from build123d import *

# Parameters (mm, degrees)
SKETCH3_W           = 41
SKETCH3_H           = 20.5
BOSS_EXTRUDE1_DEPTH = 37
SKETCH5_W           = 12
SKETCH5_H           = 8
BOSS_EXTRUDE2_DEPTH = 5
SKETCH6_R           = 1.5
CUT_EXTRUDE1_DEPTH  = 30


with BuildPart() as part:
    # Sketch3 → Boss-Extrude1 (new body)
    with BuildSketch(Plane(origin=(0, 0, 0), x_dir=(1, 0, 0), z_dir=(0, 1, 0))):
        with Locations((20.5, 10.25)):
            Rectangle(SKETCH3_W, SKETCH3_H)
    extrude(amount=BOSS_EXTRUDE1_DEPTH)

    # Sketch5 → Boss-Extrude2 (add)
    with BuildSketch(Plane(origin=(0, 37, 0), x_dir=(1, 0, 0), z_dir=(0, 1, 0))):
        with Locations((31.406806077, 9.876249369)):
            Rectangle(SKETCH5_W, SKETCH5_H)
    extrude(amount=BOSS_EXTRUDE2_DEPTH)

    # Sketch6 → Cut-Extrude1 (cut)
    with BuildSketch(Plane(origin=(0, 42, 0), x_dir=(1, 0, 0), z_dir=(0, 1, 0))):
        with Locations((34.09544318, 9.783255032)):
            Circle(SKETCH6_R)
    extrude(amount=-CUT_EXTRUDE1_DEPTH, mode=Mode.SUBTRACT)


solid = part.part
Check sheet for the modelled part. Datum: model origin and axes. Units: mm. A direction names the side the tool comes from. Give positions to 0.01 mm unless a question says otherwise; leave off trailing zeros. Loops run counter-clockwise (first coordinate to the right, second up) from the corner with the lowest first, then second, coordinate; pieces in that order, holes last. Notation, with made-up numbers: M -4.75,8.5 L 17.25,8.5 A20 ccw 17.25,24.5 Z; hole C 50.25,72 d1. An arc over 180 degrees is marked long. Use a Markdown table: item, result. Add a question column.
Q1. Scan lines: line 1 along X through (y, z) = (39, -12); line 2 along Y through (x, z) = (10, -14); line 3 along Z through (x, y) = (33.5, 18). Record each from-to range of solid material in increasing order. Write a range as [from, to].
Q2. Sectioned sample at B-B, the plane z = -13.25. Record the cut outline in (x, y).
Q3. Sectioned sample at D-D, the plane x = 3. Record the cut outline in (y, z), then the cut area to 4 significant figures.
Q4. Sectioned sample at C-C, the plane y = 38.5. Record the cut outline in (x, z).
Q5. Tool access check on faces 1 (the flat face through (31, 39, -13.876)), 2 (the flat face through (37.407, 39, -10)), 3 (the flat face through (34, 12, -10)), 4 (the flat face through (31, 39, -5.876)). Record the directions out of +Z, -Z, +X, -X, +Y, -Y that give a thin tool (end or side, any length) a straight path to the whole face; none if there is none.
Q6. Sectioned sample at A-A, the plane x = 30.5. Record the cut outline in (y, z).
Q7. Go/stop test with flat-tipped pins: pin 1 (1 mm diameter, centred on x = 28.5, z = -15, fed in from +Y); pin 2 (1.5 mm diameter, centred on y = 39, z = -9.5, fed in from -X); pin 3 (1.5 mm diameter, centred on y = 39, z = -11.5, fed in from +X). Record where each tip stops, or that it passes through.
Q8. Mould release check, pull along Z, two halves, no side actions. Record for faces 5 (the cylindrical face through (32.905, 27.21, -8.871)), 6 (the flat face through (20, 18, 0)), 7 (the flat face through (25.407, 39, -10)): pulls with the +Z half, pulls with the -Z half, needs draft (parallel to the pull), parting line crosses it, or undercut.
Verdict:
| question | item | result |
|---|---|---|
| 1 | line 1 | [25.41, 37.41] |
| 1 | line 2 | [0, 37] |
| 1 | line 3 | [-20.5, -11.16], [-8.41, 0] |
| 2 | outline | M 0,0 L 41,0 L 41,37 L 37.41,37 L 37.41,42 L 25.41,42 L 25.41,37 L 0,37 Z |
| 3 | outline | M 0,-20.5 L 37,-20.5 L 37,0 L 0,0 Z |
| 3 | area | 758.5 mm^2 |
| 4 | outline | M 25.41,-13.88 L 37.41,-13.88 L 37.41,-5.88 L 25.41,-5.88 Z; hole C 34.1,-9.78 d3 |
| 5 | face 1 | -Z, +X, -X, +Y |
| 5 | face 2 | +Z, -Z, +X, +Y |
| 5 | face 3 | +Y |
| 5 | face 4 | +Z, +X, -X, +Y |
| 6 | outline | M 0,-20.5 L 37,-20.5 L 37,-13.88 L 42,-13.88 L 42,-5.88 L 37,-5.88 L 37,0 L 0,0 Z |
| 7 | pin 1 | y = 37 |
| 7 | pin 2 | x = 25.41 |
| 7 | pin 3 | x = 37.41 |
| 8 | face 5 | undercut |
| 8 | face 6 | pulls with the +Z half |
| 8 | face 7 | needs draft |
